from build123d import *

# Parameters (mm, degrees)
F1_DEPTH = 5.08
F2_R     = 22.04107
F2_R_2   = 19.11099
F3_DEPTH = 3.048
F4_W     = 19.304385
F4_H     = 2.671048
F5_DEPTH = 3.81
F4_W_2   = 41.644052
F6_DEPTH = 3.048


with BuildPart() as f1:
    # F0 (on Top) → F1 (new body)
    with BuildSketch(Plane.XY):
        Polygon((50.798323, -0.41276), (-25.041701, 44.199018), (-25.756622, -43.786259), align=None)
        Polygon((43.80493, -0.616712), (-22.436553, -37.627826), (-21.368377, 38.244538), align=None, mode=Mode.SUBTRACT)
    extrude(amount=F1_DEPTH)

    # F2 (on Top) → F3 (join)
    with BuildSketch(Plane.XY):
        Circle(F2_R)
        Circle(F2_R_2, mode=Mode.SUBTRACT)
    extrude(amount=F3_DEPTH)

    # F4 (on Top) → F5 (join)
    with BuildSketch(Plane.XY):
        with Locations((-9.652192, -1.335524)):
            Rectangle(F4_W, F4_H)
    extrude(amount=F5_DEPTH)

    # F4 (on Top) → F6 (join)
    with BuildSketch(Plane.XY):
        with Locations((20.822026, -1.335524)):
            Rectangle(F4_W_2, F4_H)
        with Locations((-9.652192, -1.335524)):
            Rectangle(F4_W, F4_H)
    extrude(amount=F6_DEPTH)


solid = f1.part
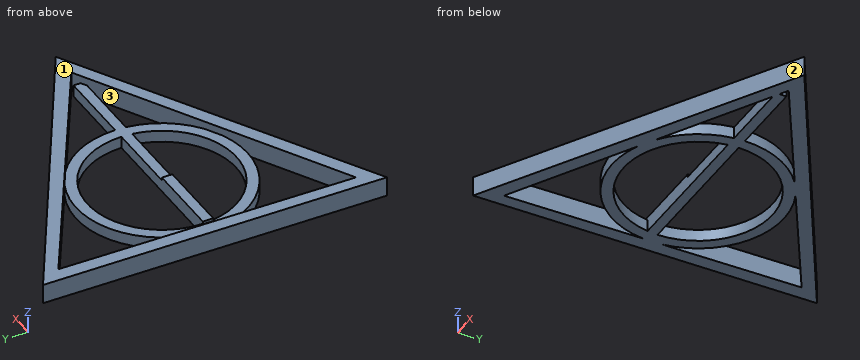
CAD build for the part. Positions are in the model's coordinates, mm. Face numbers are marked on the shaded views. Give positions to 0.01 mm unless a question says otherwise; leave off trailing zeros. Write each loop counter-clockwise with the first axis right and the second up, starting at its lowest first coordinate (ties: lowest second). Pieces come first, ordered by that corner, then holes. Notation, with made-up numbers: (-4.5, -28.75) -> (-0.5, -28.75) arc R11 cw to (-0.5, -11.75) -> close; hole circle Ø9 at (71, 25). An arc over 180 degrees is marked (long way). Return JSON: item names as keys, results as strings.
Item 1: Band-saw the part on A-A (x = 4). List the corners of the cut face in (y, z).
Answer below:
{"outline": "(-26.93, 0) -> (-22.86, 0) -> (-22.86, 5.08) -> (-26.93, 5.08) -> close; (-21.68, 0) -> (-18.69, 0) -> (-18.69, 3.05) -> (-21.68, 3.05) -> close; (-2.67, 0) -> (0, 0) -> (0, 3.05) -> (-2.67, 3.05) -> close; (18.69, 0) -> (21.68, 0) -> (21.68, 3.05) -> (18.69, 3.05) -> close; (23.12, 0) -> (27.12, 0) -> (27.12, 5.08) -> (23.12, 5.08) -> close"}
Item 2: Band-saw the part on C-C (y = -34.5). List the corners of the cut face in (x, z).
Answer below:
{"outline": "(-25.68, 0) -> (-22.39, 0) -> (-22.39, 5.08) -> (-25.68, 5.08) -> close; (-16.84, 0) -> (-9.37, 0) -> (-9.37, 5.08) -> (-16.84, 5.08) -> close"}
Item 3: Drill centre lines: probe 1 along X at (y, z) = (-9, 1.4); probe 2 along X at (y, z) = (-14, 1.6); probe 3 along Y at (x, z) = (-12, 1.4). Where is each one in solid material? Low to high.
Answer below:
{"probe 1": "x = -25.47 to -22.03, -20.12 to -16.86, 16.86 to 20.12, 28.8 to 35.64", "probe 2": "x = -25.51 to -22.1, -17.02 to -13.01, 13.01 to 17.02, 19.85 to 26.82", "probe 3": "y = -35.99 to -31.8, -18.49 to -14.87, -2.67 to 0, 14.87 to 18.49, 32.66 to 36.53"}
Item 4: Band-saw the part on D-D (y = -9). List the corners of the cut face in (x, z).
Answer below:
{"outline": "(-25.47, 0) -> (-22.03, 0) -> (-22.03, 5.08) -> (-25.47, 5.08) -> close; (-20.12, 0) -> (-16.86, 0) -> (-16.86, 3.05) -> (-20.12, 3.05) -> close; (16.86, 0) -> (20.12, 0) -> (20.12, 3.05) -> (16.86, 3.05) -> close; (28.8, 0) -> (35.64, 0) -> (35.64, 5.08) -> (28.8, 5.08) -> close"}
Item 5: Drop flat-ended pins along their axis: pin 1 (1 mm diameter, centred on x = 25, z = 1.5, fed in from -Y); pin 2 (1.9 mm diameter, centred on x = -1.5, z = 1, fed in from -Y); pin 3 (1.5 mm diameter, centred on y = -1, z = 1.5, fed in from +X). Give the stop position or say it passes through.
Answer below:
{"pin 1": "stops at y = -15.31", "pin 2": "stops at y = -30.58", "pin 3": "stops at x = 50.8"}
Item 6: Band-saw the part on B-B (y = 15.5). List the corners of the cut face in (x, z), then the cut area to 3 significant figures.
Answer below:
{"outline": "(-25.27, 0) -> (-21.69, 0) -> (-21.69, 5.08) -> (-25.27, 5.08) -> close; (-15.67, 0) -> (-11.18, 0) -> (-11.18, 3.05) -> (-15.67, 3.05) -> close; (11.18, 0) -> (15.67, 0) -> (15.67, 3.05) -> (11.18, 3.05) -> close; (16.78, 0) -> (23.75, 0) -> (23.75, 5.08) -> (16.78, 5.08) -> close", "area": "81.0 mm2"}
Item 7: Two-plate mould, pull along Y, no slides. Class the marked faces 1, 2 and 3: +Y half, -Y half, draft (parallel to the pull), parting line (faces both ways), or undercut.
Answer below:
{"face 1": "draft", "face 2": "-Y half", "face 3": "undercut"}
